Could you check a few things on this model? Use its own coordinates, in mm. Give positions to 0.01 mm unless a question says otherwise; leave off trailing zeros. Loops run counter-clockwise (first coordinate to the right, second up) from the corner with the lowest first, then second, coordinate; pieces in that order, holes last. Notation, with made-up numbers: (28, 44.5) - (36, 44.5) arc R23 ccw to (36, 73.5) - close; hole circle Ø8 at (54, -12). An arc over 180 degrees is marked (long way). Use CSV: the item, a comma, the result in double quotes.
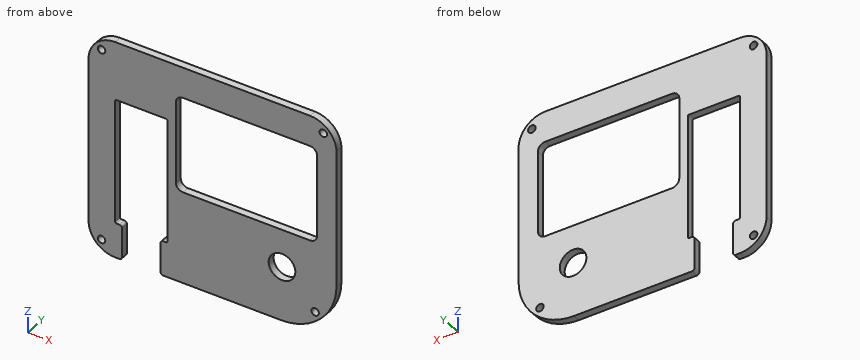
from build123d import *

# Parameters (mm, degrees)
SKETCH2_R           = 5.5
SKETCH2_R_2         = 1.55
BOSS_EXTRUDE1_DEPTH = 3.048


with BuildPart() as part:
    # Sketch2 → Boss-Extrude1 (new body)
    with BuildSketch(Plane(origin=(0, 0, 0), x_dir=(1, 0, 0), z_dir=(0, 1, 0))):
        with BuildLine():
            Line((3, -6.84), (3, -57.34))
            ThreePointArc((3, -57.34), (3.146446609, -57.693553391), (3.5, -57.84))
            Line((3.5, -57.84), (24, -57.84))
            ThreePointArc((24, -57.84), (24.353553391, -57.693553391), (24.5, -57.34))
            Line((24.5, -57.34), (24.5, -6.84))
            ThreePointArc((24.5, -6.84), (24.353553391, -6.486446609), (24, -6.34))
            Line((24, -6.34), (22.75, -6.34))
            ThreePointArc((22.75, -6.34), (22.042893219, -6.047106781), (21.75, -5.34))
            Line((21.75, -5.34), (21.75, 7))
            ThreePointArc((21.75, 7), (22.042893219, 7.707106781), (22.75, 8))
            Line((22.75, 8), (71.45, 8))
            ThreePointArc((71.45, 8), (87.628603154, 1.298603154), (94.33, -14.88))
            Line((94.33, -14.88), (94.33, -71.310147445))
            ThreePointArc((94.33, -71.310147445), (90.950189058, -78.782657675), (83.340051803, -81.84))
            Line((83.340051803, -81.84), (3, -81.84))
            ThreePointArc((3, -81.84), (-4.778174593, -78.618174593), (-8, -70.84))
            Line((-8, -70.84), (-8, -3))
            ThreePointArc((-8, -3), (-4.778174593, 4.778174593), (3, 8))
            Line((3, 8), (4.75, 8))
            ThreePointArc((4.75, 8), (5.457106781, 7.707106781), (5.75, 7))
            Line((5.75, 7), (5.75, -5.34))
            ThreePointArc((5.75, -5.34), (5.457106781, -6.047106781), (4.75, -6.34))
            Line((4.75, -6.34), (3.5, -6.34))
            ThreePointArc((3.5, -6.34), (3.146446609, -6.486446609), (3, -6.84))
        make_face()
        with Locations(Location((71.83, -14.33, 0), (0, 0, 90))):
            Circle(SKETCH2_R, mode=Mode.SUBTRACT)
        with Locations(Location((-2.656854249, 2.656854249, 0), (0, 0, 90))):
            Circle(SKETCH2_R_2, mode=Mode.SUBTRACT)
        with Locations(Location((85.50728281, -0.82271719, 0), (0, 0, 90))):
            Circle(SKETCH2_R_2, mode=Mode.SUBTRACT)
        with Locations(Location((88.858862501, -76.631761762, 0), (0, 0, 90))):
            Circle(SKETCH2_R_2, mode=Mode.SUBTRACT)
        with Locations(Location((-2.656854249, -76.496854249, 0), (0, 0, 90))):
            Circle(SKETCH2_R_2, mode=Mode.SUBTRACT)
        with BuildLine():
            Line((28, -66.24), (28, -32.84))
            ThreePointArc((28, -32.84), (28.878679656, -30.718679656), (31, -29.84))
            Line((31, -29.84), (83.33, -29.84))
            ThreePointArc((83.33, -29.84), (85.451320344, -30.718679656), (86.33, -32.84))
            Line((86.33, -32.84), (86.33, -66.24))
            ThreePointArc((86.33, -66.24), (85.451320344, -68.361320344), (83.33, -69.24))
            Line((83.33, -69.24), (31, -69.24))
            ThreePointArc((31, -69.24), (28.878679656, -68.361320344), (28, -66.24))
        make_face(mode=Mode.SUBTRACT)
    extrude(amount=BOSS_EXTRUDE1_DEPTH)


solid = part.part
1) Suppose I cut it at C-C (z = 59). Please give me the cut outline in (x, y).
Answer below:
outline,"(-8, 0) - (28, 0) - (28, 3.05) - (-8, 3.05) - close; (86.33, 0) - (94.33, 0) - (94.33, 3.05) - (86.33, 3.05) - close"
2) Suppose I cut it at B-B (z = 11). Please give me the cut outline in (x, y), plus the area to 3 significant figures.
Answer below:
outline,"(-8, 0) - (3, 0) - (3, 3.05) - (-8, 3.05) - close; (24.5, 0) - (67.45, 0) - (67.45, 3.05) - (24.5, 3.05) - close; (76.21, 0) - (94, 0) - (94, 3.05) - (76.21, 3.05) - close"
area,"219 mm2"
3) I'm going to push flat-ended pins straight in: P1, Ø3, axis at x = 85.51, z = 0.82, coming from the +Y side; P2, Ø0.9, axis at y = 1, z = 2, coming from the +X side. Where does each tip first touch, or does it pass through?
Answer below:
P1,"passes through"
P2,"stops at x = 90.66"
4) Suppose I cut it at D-D (y = 2.2). State how many separate pieces and enclosed holes the cut face has, plus the area to 3 significant figures.
Answer below:
separate pieces,"1"
enclosed holes,"6"
area,"5,250 mm2"
5) Suppose I cut it at A-A (x = 41.5). Please give me the cut outline in (y, z), plus the area to 3 significant figures.
Answer below:
outline,"(0, -8) - (3.05, -8) - (3.05, 29.84) - (0, 29.84) - close; (0, 69.24) - (3.05, 69.24) - (3.05, 81.84) - (0, 81.84) - close"
area,"154 mm2"
6) I need wall thicknesses on line 1 along X through (y, z) = (2.85, 35.5); line 2 along X through (y, z) = (2.6, 14.5); line 3 along Z through (x, y) = (35, 1). Which ranges of each line are inside material? Lowest first, please.
Answer below:
line 1,"x = -8 to 3, 24.5 to 28, 86.33 to 94.33"
line 2,"x = -8 to 3, 24.5 to 66.33, 77.33 to 94.33"
line 3,"z = -8 to 29.84, 69.24 to 81.84"
